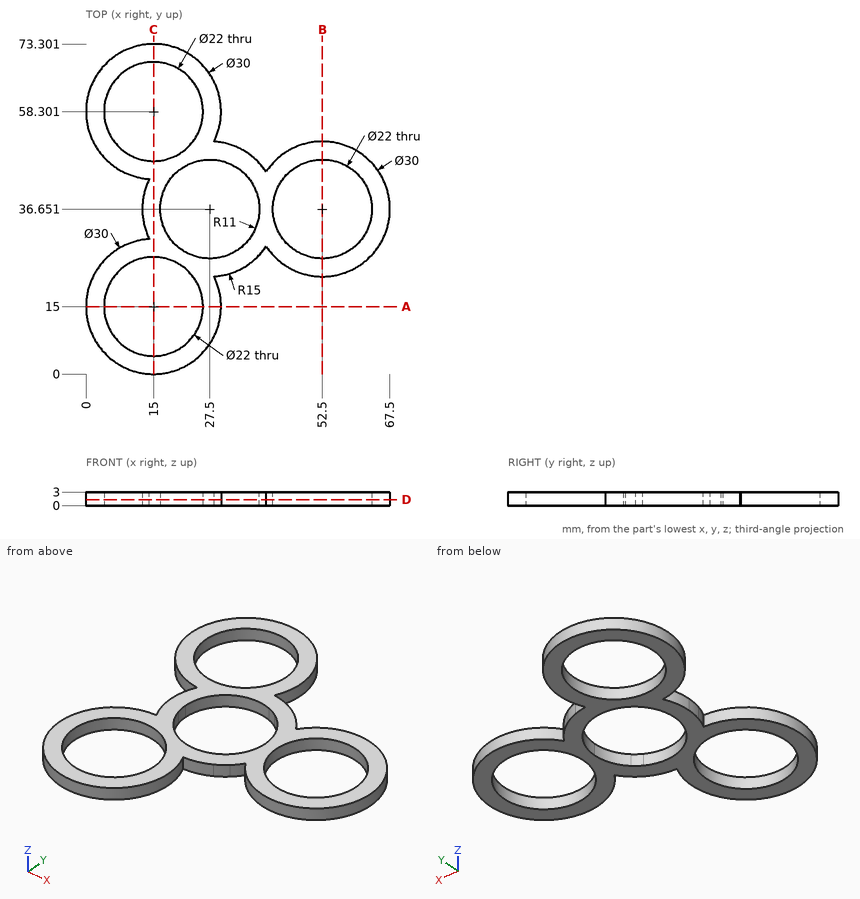
Geometry check sheet. Reference: drawing and pictorial views, mm from the part's lowest x, y, z. Give positions to 0.01 mm unless a question says otherwise; leave off trailing zeros. Write each loop counter-clockwise with the first axis right and the second up, starting at its lowest first coordinate (ties: lowest second). Pieces come first, ordered by that corner, then holes. Notation, with made-up numbers: M -31,6.25 L 7,6.25 A16 cw 7,17.25 Z; hole C 32,88 d8. An arc over 180 degrees is marked long. Put each result on its own line as item: value. Start each with the question number.
1. Section check A-A (y = 15). Record the cut outline in (x, z), and give its area (3 significant figures).
2. Scan lines: line 1 along Y through (x, z) = (15, 2.25); line 2 along Y through (x, z) = (52.5, 1.2); line 3 along X through (y, z) = (50, 2.35) (1 decimal). Record each from-to range of solid material in increasing order. Write a range as [from, to].
3. Section check D-D (z = 1.3). Give the number of separate pieces and of enclosed holes in the cut face, and give its area (3 significant figures).
4. Go/stop test with flat-tipped pins: pin 1 Ø1 at (y, z) = (39.5, 2) entering from +X (1 decimal); pin 2 Ø1 at (y, z) = (52, 1) entering from -X; pin 3 Ø20 at (x, y) = (52.5, 36.65) entering from -Z. Record where each tip stops, or that it passes through.
5. Section check C-C (x = 15). Record the cut outline in (y, z).
6. Section check B-B (x = 52.5). Record the cut outline in (y, z).
Answer list:
1. outline: M 0,0 L 4,0 L 4,3 L 0,3 Z; M 26,0 L 30,0 L 30,3 L 26,3 Z
1. area: 24.0 mm2
2. line 1: [0, 4], [26, 47.3], [69.3, 73.3]
2. line 2: [21.65, 25.65], [47.65, 51.65]
2. line 3: [2.5, 7.8], [22.2, 34.3], [45.7, 59.3]
3. separate pieces: 1
3. enclosed holes: 4
3. area: 1,140 mm2
4. pin 1: x = 67.3
4. pin 2: x = 1.17
4. pin 3: through
5. outline: M 0,0 L 4,0 L 4,3 L 0,3 Z; M 26,0 L 47.3,0 L 47.3,3 L 26,3 Z; M 69.3,0 L 73.3,0 L 73.3,3 L 69.3,3 Z
6. outline: M 21.65,0 L 25.65,0 L 25.65,3 L 21.65,3 Z; M 47.65,0 L 51.65,0 L 51.65,3 L 47.65,3 Z
